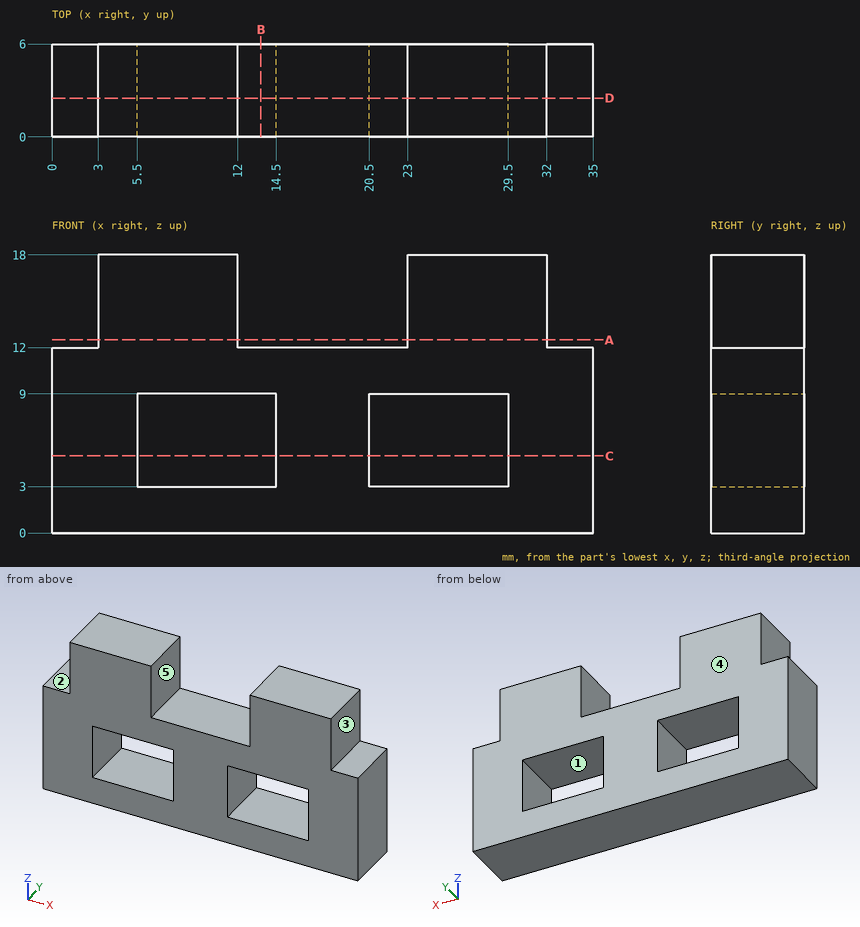
Answer from the drawing. Dimensions are ordinates in mm from the lowest x, y and z of the part. A direction names the side the tool comes from. Round coordinates to 2 decimals unless told otherwise and drop trailing zeros. Order: outer loops, then holes, each group sorted by start corner. A loop starts at its lowest first (then second) coordinate and runs counter-clockwise, first axis right, second up.
1) The part is cut by section D-D on y = 2.5. Write down the section's boundary in (x, z), plus the area to 3 significant figures.
2) The part is cut by section C-C on z = 5. Write down the section's boundary in (x, y), plus the area to 3 significant figures.
3) The part is cut by section B-B on x = 13.5. Write down the section's boundary in (y, z), plus the area to 3 significant figures.
4) For the marked faces 1, 2, 3, 4 and 5, determine the directions among +Z, -Z, +X, -X, +Y, -Y from which every point of the face is accessible in a straight line to the end or side of a thin tool.
5) Flat-ended cylindrical pins translate along their axes: pin 1 (3 mm diameter, centred on x = 25, y = 1.5, fed in from -Z); pin 2 (3 mm diameter, centred on y = 4, z = 16.5, fed in from -X); pin 3 (1.5 mm diameter, centred on x = 33, y = 3.5, fed in from +Z). Find the tip coordinate at first contact, or state that the pin passes through.
6) Straight lines are drawn through the part: L1, parallel to X at y = 0.3, z = 8.75; L2, parallel to Z at x = 7, y = 2.05; L3, parallel to X at y = 4.7, z = 15.75. For each, find the intervals that lie inside material, in ascending order.
7) The part is cut by section A-A on z = 12.5. Write down the section's boundary in (x, y), plus the area to 3 significant figures.
Resolved:
1. outline: (0, 0) - (35, 0) - (35, 12) - (32, 12) - (32, 18) - (23, 18) - (23, 12) - (12, 12) - (12, 18) - (3, 18) - (3, 12) - (0, 12) - close; hole (5.5, 3) - (14.5, 3) - (14.5, 9) - (5.5, 9) - close; hole (20.5, 3) - (29.5, 3) - (29.5, 9) - (20.5, 9) - close
1. area: 420 mm2
2. outline: (0, 0) - (5.5, 0) - (5.5, 6) - (0, 6) - close; (14.5, 0) - (20.5, 0) - (20.5, 6) - (14.5, 6) - close; (29.5, 0) - (35, 0) - (35, 6) - (29.5, 6) - close
2. area: 102 mm2
3. outline: (0, 0) - (6, 0) - (6, 3) - (0, 3) - close; (0, 9) - (6, 9) - (6, 12) - (0, 12) - close
3. area: 36.0 mm2
4. face 1: +Y, -Y
4. face 2: +Z, -X, +Y, -Y
4. face 3: +Z, +X, +Y, -Y
4. face 4: +Z, -Z, +X, -X, +Y
4. face 5: +Z, +Y, -Y
5. pin 1: stops at z = 0
5. pin 2: stops at x = 3
5. pin 3: stops at z = 12
6. L1: x = 0 to 5.5, 14.5 to 20.5, 29.5 to 35
6. L2: z = 0 to 3, 9 to 18
6. L3: x = 3 to 12, 23 to 32
7. outline: (3, 0) - (12, 0) - (12, 6) - (3, 6) - close; (23, 0) - (32, 0) - (32, 6) - (23, 6) - close
7. area: 108 mm2
